Could you check a few things on this model? Use its own coordinates, in mm. A direction names the side the tool comes from. Round coordinates to 2 decimals unless told otherwise and drop trailing zeros. Order: outer loops, then holes, each group sorted by start corner. A loop starts at its lowest first (then second) coordinate and runs counter-clockwise, first axis right, second up. Notation, with made-up numbers: (22, 30.25) - (77, 30.25) arc R25 ccw to (77, 67.25) - close; hole circle Ø11 at (35, -8.75). An arc over 180 degrees is marked (long way). Return JSON: item names as keys, results as strings. Group by question number.
from build123d import *

# Parameters (mm, degrees)
F1_DEPTH = 12.7
F2_W     = 3.81
F2_H     = 25.6764874435
F3_DEPTH = 25.4
F4_R     = 1.524


with BuildPart() as f1:
    # F0 (on Top) → F1 (new body)
    with BuildSketch(Plane.XY):
        with BuildLine():
            Line((-3.81, 7.7796718605), (-3.81, -7.7796718605))
            ThreePointArc((-3.81, -7.7796718605), (0, -18.923), (3.81, -7.7796718605))
            Line((3.81, -7.7796718605), (3.81, 7.7796718605))
            ThreePointArc((3.81, 7.7796718605), (0, 18.923), (-3.81, 7.7796718605))
        make_face()
    extrude(amount=F1_DEPTH)

    # F2 (on face) → F3 (cut)
    with BuildSketch(Plane(origin=(0, 0, 0), x_dir=(1, 0, 0), z_dir=(0, 0, -1))):
        with Locations((0, -16.6482437217)):
            Rectangle(F2_W, F2_H)
        with Locations((0, 16.6482437217)):
            Rectangle(F2_W, F2_H)
    extrude(amount=-F3_DEPTH, mode=Mode.SUBTRACT)

    # F4
    f4_edges = [f1.edges().sort_by_distance(p)[0] for p in [
        (1.905, 3.81, 6.35),
        (-1.905, 3.81, 6.35),
        (1.905, -3.81, 6.35),
        (-1.905, -3.81, 6.35),
    ]]
    fillet(f4_edges, radius=F4_R)


solid = f1.part
1) We'd pull the mould along Y, two halves only. Please class faces 5 (the cylindrical face through (1.4, 4.2, 6.4)), 6 (the cylindrical face through (-6.11, 13.87, 6.26)), 7 (the flat face through (1.905, -12, 6)): +Y half, -Y half, draft (parallel to the pull), parting line (faces both ways), or undercut.
2) Will these pins go through, and if not, where does the flat tip stop? pin 1 (4 mm diameter, centred on y = -10, z = 6.5, fed in from -X); pin 2 (0.8 mm diameter, centred on x = 0, z = 9.5, fed in from -Y); pin 3 (4 mm diameter, centred on y = -2, z = 6.5, fed in from -X).
3) If I drill on line 1 along X through (y, z) = (-9.5, 2.5) (3 decimals); line 2 along X through (y, z) = (6, 2.5) (3 decimals); line 3 along Y through (x, z) = (-4, 5.75), over which ranges is the centre line in solid material (lowest first)? Write a range as from..to.
4) For faces 1 (the flat face through (3.81, 0, 6)), 2 (the flat face through (-3.81, 0, 6)), 3 (the flat face through (-1.905, -12, 6)), 4 (the flat face through (1.905, 12, 6)), which set-ups out of +Z, -Z, +X, -X, +Y, -Y let a thin tool reach every point of the face, with its end or its side?
5) I want a section at B-B, the plane y = 9. List the corners of the cut face in (x, z) for me (3 decimals), plus the area to 3 significant figures.
6) I want a section at A-A, the plane x = -4.75. List the corners of the cut face in (y, z) for me, plus the area to 3 significant figures.
7) I want a section at C-C, the plane z = 8.25. List the corners of the cut face in (x, y) for me (3 decimals).
8) I want a section at D-D, the plane y = -3. List the corners of the cut face in (x, z) for me.
Outcome:
{
 "1": {"face 5": "+Y half", "face 6": "undercut", "face 7": "draft"},
 "2": {"pin 1": "x = -6.18", "pin 2": "y = -3.81", "pin 3": "x = -3.81"},
 "3": {"line 1": "-5.337..-1.905, 1.905..5.337", "line 2": "-3.81..-1.905, 1.905..3.81", "line 3": "-17.47..-7.93, 7.93..17.47"},
 "4": {"face 1": "+Z, -Z, +X", "face 2": "+Z, -Z, -X", "face 3": "+Z, -Z, -Y", "face 4": "+Z, -Z, +Y"},
 "5": {"outline": "(-5.004, 0) - (-1.905, 0) - (-1.905, 12.7) - (-5.004, 12.7) - close; (1.905, 0) - (5.004, 0) - (5.004, 12.7) - (1.905, 12.7) - close", "area": "78.7 mm^2"},
 "6": {"outline": "(-16.72, 0) - (-8.68, 0) - (-8.68, 12.7) - (-16.72, 12.7) - close; (8.68, 0) - (16.72, 0) - (16.72, 12.7) - (8.68, 12.7) - close", "area": "204 mm^2"},
 "7": {"outline": "(-3.81, -7.78) arc R6.223 ccw to (-1.905, -18.624) - (-1.905, -5.334) arc R1.524 cw to (-0.381, -3.81) - (0.381, -3.81) arc R1.524 cw to (1.905, -5.334) - (1.905, -18.624) arc R6.223 ccw to (3.81, -7.78) - (3.81, 7.78) arc R6.223 ccw to (1.905, 18.624) - (1.905, 5.334) arc R1.524 cw to (0.381, 3.81) - (-0.381, 3.81) arc R1.524 cw to (-1.905, 5.334) - (-1.905, 18.624) arc R6.223 ccw to (-3.81, 7.78) - close"},
 "8": {"outline": "(-3.81, 0) - (3.81, 0) - (3.81, 12.7) - (-3.81, 12.7) - close"}
}
